Autodesk Fusion 360 part; units mm, degrees
sketch "Náčrt1" plane through (0, 0, 0) normal (0, 0, 1) x (1, 0, 0)
  circle A0 centre (0, 0) radius 3.5
  circle A1 centre (0, 0) radius 5.3
  line L0 (3.5, 6) -> (3.5, -6)
  line L1 (5.3, 6) -> (5.3, -6)
  line L2 (3.5, 6) -> (5.3, 6)
  line L3 (3.5, -6) -> (5.3, -6)
  line L4 (-1.5, 6) -> (-1.5, 0) construction
  circle A2 centre (-3.5, 4.2426) radius 2
  circle A3 centre (-3.5, 4.2426) radius 0.2
  line L5 (-3.5, 4.2426) -> (-2.0858, 5.6569) construction
  line L6 (-3.5, 4.2426) -> (-1.5, 4.2426) construction
  circle A4 centre (-2.7222, 5.0205) radius 0.9
  circle A5 centre (3.5, 2.6665) radius 0.9
  point P0 (3.5, 0)
  dimension "d1" = 7
  dimension "d2" = 10.6
  dimension "d3" = 12
  dimension "d4" = 5
  dimension "d5" = 4
  dimension "d6" = 45
extrude "Vysunutí1" add sketch "Náčrt1" along normal blind 12 contours A0 A1 L0 A2 | A0 L0 A5 | A1 L0 A5 | L0 A5 | A1 A2 A4 | L0 A5 | A1 L0 L1 L3 | A1 L0 A5 | A1 L0 L1 L2 | A1 A3 A4 | A1 A2 A4 | A1 A4 | A1 A4
fillet "Zaoblení1" radius 0.6 2 edges at (3.5, -6, 6) (3.5, 6, 6)
fillet "Zaoblení1" radius 1 1 edges at (3.5, -3.9799, 6)
fillet "Zaoblení1" radius 0.4 1 edges at (3.5, 3.5665, 6)
chamfer "Zkosení2" distance 0.2 angle 45 2 faces at (4.6974, 0.0779, 0) (4.6974, 0.0779, 12)
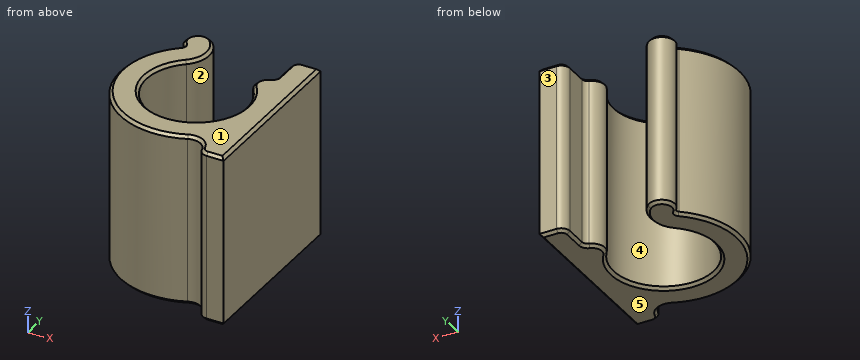
Part model, mm, in its own coordinate system. Face numbers are marked on the shaded views. A direction names the side the tool comes from. Give positions to 0.01 mm unless a question says otherwise; leave off trailing zeros. Order: outer loops, then holes, each group sorted by start corner. A loop starts at its lowest first (then second) coordinate and runs counter-clockwise, first axis right, second up. Notation, with made-up numbers: M 55,-22 L 112,-22 A18 ccw 112,-3 Z; hole C -25,73.25 d2. An arc over 180 degrees is marked long. Use a Markdown table: item, result. Add a question column.
(1) 3-axis set-ups, long thin cutter, end or side, ignore diameter. For the marked faces 1 and 2: which of +Z, -Z, +X, -X, +Y, -Y reach the whole face in a straight line?
(2) Probe line 1 along X through (y, z) = (0, 4); line 2 along X through (y, z) = (2, 1.75); line 3 along Y through (x, z) = (0, 8.75). List the from-to ranges inside material, lowest first. Write a range as [from, to].
(3) Saw through at B-B, the plane x = 0. Give the cut face in (y, z).
(4) Saw through at A-A, the plane y = 0. Give the cut face in (x, z).
(5) Drop flat-ended pins along their axis: P1, Ø1, axis at x = 0, z = 8, coming from the +Y side; P2, Ø1.2, axis at y = 4.5, z = 8.5, coming from the -X side; P3, Ø1.5, axis at x = 0, y = 3.5, coming from the -Z side; P4, Ø1, axis at x = 0.5, z = 1.5, coming from the -Y side. Give the stop position or say it passes through.
(6) Mould opens along Y. For the marked faces 3, 4 and 5 say: +Y half, -Y half, draft (parallel to the pull), parting line (faces both ways), or undercut.
Answer key:
| question | item | result |
|---|---|---|
| 1 | face 1 | +Z, +X, -X, +Y, -Y |
| 1 | face 2 | +Z, -Z |
| 2 | line 1 | [-5.3, -3.5], [3.5, 5.3] |
| 2 | line 2 | [-4.91, -2.87], [2.87, 5.3] |
| 2 | line 3 | [-5.3, -3.5] |
| 3 | outline | M -5.3,0.2 L -5.1,0 L -3.7,0 L -3.5,0.2 L -3.5,11.8 L -3.7,12 L -5.1,12 L -5.3,11.8 Z |
| 4 | outline | M -5.3,0.2 L -5.1,0 L -3.7,0 L -3.5,0.2 L -3.5,11.8 L -3.7,12 L -5.1,12 L -5.3,11.8 Z; M 3.5,0.2 L 3.7,0 L 5.1,0 L 5.3,0.2 L 5.3,11.8 L 5.1,12 L 3.7,12 L 3.5,11.8 Z |
| 5 | P1 | y = -3.46 |
| 5 | P2 | x = -3.62 |
| 5 | P3 | through |
| 5 | P4 | y = -5.3 |
| 6 | face 3 | +Y half |
| 6 | face 4 | undercut |
| 6 | face 5 | draft |
